```python
from build123d import *

# Parameters (mm, degrees)
SKETCH1_W           = 133
SKETCH1_H           = 105
BOSS_EXTRUDE1_DEPTH = 60
CUT_EXTRUDE1_START  = -2
CUT_EXTRUDE1_DEPTH  = 129
SKETCH3_R           = 42.5
CUT_EXTRUDE2_DEPTH  = 10
FILLET1_R           = 2.5
SKETCH4_W           = 50
SKETCH4_H           = 45
BOSS_EXTRUDE2_DEPTH = 6
SKETCH5_R           = 2.525
CUT_EXTRUDE3_DEPTH  = 4
BOSS_EXTRUDE3_START = 6.5
BOSS_EXTRUDE3_DEPTH = 5
BOSS_EXTRUDE4_START = 11.5
BOSS_EXTRUDE4_DEPTH = 5
CUT_EXTRUDE5_REACH  = 182.394


with BuildPart() as part:
    # Sketch1 → Boss-Extrude1 (new body)
    with BuildSketch(Plane(origin=(0, 0, 0), x_dir=(1, 0, 0), z_dir=(0, 1, 0))):
        with Locations((66.5, 52.5)):
            Rectangle(SKETCH1_W, SKETCH1_H)
    extrude(amount=BOSS_EXTRUDE1_DEPTH)

    # Sketch2 → Cut-Extrude1 (cut)
    with BuildSketch(Plane.ZY.offset(CUT_EXTRUDE1_START)):
        with BuildLine():
            Line((-99, 0), (-6, 0))
            ThreePointArc((-6, 0), (-52.5, 46.5), (-99, 0))
        make_face()
    extrude(amount=-CUT_EXTRUDE1_DEPTH, mode=Mode.SUBTRACT)

    # Sketch3 → Cut-Extrude2 (cut)
    with BuildSketch(Plane.ZY):
        with Locations((-52.5, 0)):
            Circle(SKETCH3_R)
    extrude(amount=-CUT_EXTRUDE2_DEPTH, mode=Mode.SUBTRACT)

    # Fillet1
    # the kernel refuses this fillet: 2.5 mm, written as the material it takes off along each edge
    with BuildSketch(Plane(origin=(130.5, 57.5, -102.5), x_dir=(0, 1, 0), z_dir=(1, 0, 0))) as fillet1_piece_1_section:
        Polygon((0, 0), (FILLET1_R * 1.02, 0), (FILLET1_R * 1.02, -FILLET1_R * 1.02), (0, -FILLET1_R * 1.02), align=None)
    fillet1_piece_1 = extrude(amount=FILLET1_R * 1.02, mode=Mode.PRIVATE)
    fillet1_piece_1 = fillet1_piece_1 - Plane(origin=(130.5, 57.5, -102.5), x_dir=(0, -0.7071067811865475, 0.7071067811865475), z_dir=(1, 0, 0)) * Sphere(FILLET1_R, mode=Mode.PRIVATE)
    add(fillet1_piece_1, mode=Mode.SUBTRACT)
    with BuildSketch(Plane(origin=(2.5, 57.5, -102.5), x_dir=(0, 1, 0), z_dir=(-1, 0, 0))) as fillet1_piece_2_section:
        Polygon((0, 0), (FILLET1_R * 1.02, 0), (FILLET1_R * 1.02, FILLET1_R * 1.02), (0, FILLET1_R * 1.02), align=None)
    fillet1_piece_2 = extrude(amount=FILLET1_R * 1.02, mode=Mode.PRIVATE)
    fillet1_piece_2 = fillet1_piece_2 - Plane(origin=(2.5, 57.5, -102.5), x_dir=(0, -0.7071067811865475, 0.7071067811865475), z_dir=(-1, 0, 0)) * Sphere(FILLET1_R, mode=Mode.PRIVATE)
    add(fillet1_piece_2, mode=Mode.SUBTRACT)
    with BuildSketch(Plane(origin=(130.5, 57.5, -2.5), x_dir=(1, 0, 0), z_dir=(0, 0, 1))) as fillet1_piece_3_section:
        Polygon((0, 0), (FILLET1_R * 1.02, 0), (FILLET1_R * 1.02, FILLET1_R * 1.02), (0, FILLET1_R * 1.02), align=None)
    fillet1_piece_3 = extrude(amount=FILLET1_R * 1.02, mode=Mode.PRIVATE)
    fillet1_piece_3 = fillet1_piece_3 - Plane(origin=(130.5, 57.5, -2.5), x_dir=(-0.7071067811865475, -0.7071067811865475, 0), z_dir=(0, 0, 1)) * Sphere(FILLET1_R, mode=Mode.PRIVATE)
    add(fillet1_piece_3, mode=Mode.SUBTRACT)
    with BuildSketch(Plane(origin=(2.5, 57.5, -2.5), x_dir=(-1, 0, 0), z_dir=(0, 0, 1))) as fillet1_piece_4_section:
        Polygon((0, 0), (FILLET1_R * 1.02, 0), (FILLET1_R * 1.02, -FILLET1_R * 1.02), (0, -FILLET1_R * 1.02), align=None)
    fillet1_piece_4 = extrude(amount=FILLET1_R * 1.02, mode=Mode.PRIVATE)
    fillet1_piece_4 = fillet1_piece_4 - Plane(origin=(2.5, 57.5, -2.5), x_dir=(0.7071067811865475, -0.7071067811865475, 0), z_dir=(0, 0, 1)) * Sphere(FILLET1_R, mode=Mode.PRIVATE)
    add(fillet1_piece_4, mode=Mode.SUBTRACT)
    with BuildSketch(Plane(origin=(130.5, 60, -105), x_dir=(0, 0, 1), z_dir=(-1, 0, 0))) as fillet1_piece_5:
        with BuildLine():
            CenterArc((FILLET1_R, -FILLET1_R), FILLET1_R, 90, 90)
            Line((0, -FILLET1_R), (0, 0))
            Line((0, 0), (FILLET1_R, 0))
        make_face()
    extrude(amount=128, mode=Mode.SUBTRACT)
    with BuildSketch(Plane(origin=(133, 60, -2.5), x_dir=(0, -1, 0), z_dir=(0, 0, -1)), Plane(origin=(0, 60, -102.5), x_dir=(0, -1, 0), z_dir=(0, 0, 1))) as fillet1_piece_6:
        with BuildLine():
            CenterArc((FILLET1_R, FILLET1_R), FILLET1_R, 180, 90)
            Line((0, FILLET1_R), (0, 0))
            Line((0, 0), (FILLET1_R, 0))
        make_face()
    extrude(amount=100, mode=Mode.SUBTRACT)
    with BuildSketch(Plane(origin=(2.5, 60, 0), x_dir=(0, -1, 0), z_dir=(1, 0, 0))) as fillet1_piece_7:
        with BuildLine():
            CenterArc((FILLET1_R, FILLET1_R), FILLET1_R, 180, 90)
            Line((0, FILLET1_R), (0, 0))
            Line((0, 0), (FILLET1_R, 0))
        make_face()
    extrude(amount=128, mode=Mode.SUBTRACT)
    with BuildSketch(Plane(origin=(133, -6.25, 0), x_dir=(-1, 0, 0), z_dir=(0, 1, 0)), Plane(origin=(133, -6.25, -105), x_dir=(0, 0, 1), z_dir=(0, 1, 0))) as fillet1_piece_8:
        with BuildLine():
            CenterArc((FILLET1_R, -FILLET1_R), FILLET1_R, 90, 90)
            Line((0, -FILLET1_R), (0, 0))
            Line((0, 0), (FILLET1_R, 0))
        make_face()
    extrude(amount=63.75, mode=Mode.SUBTRACT)
    with BuildSketch(Plane(origin=(133, 0, 6.25), x_dir=(0, 1, 0), z_dir=(0, 0, -1))) as fillet1_piece_9:
        with BuildLine():
            CenterArc((FILLET1_R, -FILLET1_R), FILLET1_R, 90, 90)
            Line((0, -FILLET1_R), (0, 0))
            Line((0, 0), (FILLET1_R, 0))
        make_face()
    extrude(amount=117.5, mode=Mode.SUBTRACT)
    with BuildSketch(Plane(origin=(0, -6.25, -105), x_dir=(0, 0, 1), z_dir=(0, 1, 0)), Plane(origin=(0, -6.25, 0), x_dir=(1, 0, 0), z_dir=(0, 1, 0))) as fillet1_piece_10:
        with BuildLine():
            CenterArc((FILLET1_R, FILLET1_R), FILLET1_R, 180, 90)
            Line((0, FILLET1_R), (0, 0))
            Line((0, 0), (FILLET1_R, 0))
        make_face()
    extrude(amount=63.75, mode=Mode.SUBTRACT)
    with BuildSketch(Plane(origin=(0, 0, -16.25), x_dir=(0, 1, 0), z_dir=(0, 0, 1)), Plane(origin=(0, 0, -111.25), x_dir=(0, 1, 0), z_dir=(0, 0, 1))) as fillet1_piece_11:
        with BuildLine():
            CenterArc((FILLET1_R, -FILLET1_R), FILLET1_R, 90, 90)
            Line((0, -FILLET1_R), (0, 0))
            Line((0, 0), (FILLET1_R, 0))
        make_face()
    extrude(amount=22.5, mode=Mode.SUBTRACT)
    with BuildSketch(Plane(origin=(0, 0, -52.5), x_dir=(0, -0.14381889116089097, 0.9896040251258337), z_dir=(0, -0.9896040251258337, -0.14381889116089097))) as fillet1_piece_12:
        with BuildLine():
            CenterArc((44.949489743, -2.5), FILLET1_R, 90, 78.463040967)
            Line((42.5, -2), (42.5, 0))
            Line((42.5, 0), (44.949489743, 0))
        make_face()
    revolve(axis=Axis((0, 0, -52.5), (-1, 0, 0)), revolution_arc=196.537779553, mode=Mode.SUBTRACT)

    # Sketch4 → Boss-Extrude2 (add)
    with BuildSketch(Plane(origin=(0, 60, 0), x_dir=(1, 0, 0), z_dir=(0, 1, 0))):
        with Locations((66.5, 52.5)):
            Rectangle(SKETCH4_W, SKETCH4_H)
    extrude(amount=BOSS_EXTRUDE2_DEPTH)

    # Sketch5 → Cut-Extrude3 (cut)
    with BuildSketch(Plane(origin=(0, 66, 0), x_dir=(1, 0, 0), z_dir=(0, 1, 0))):
        with Locations(Location((47.5, 68.5, 0), (0, 0, 270))):
            Circle(SKETCH5_R)
        with Locations(Location((85.5, 68.5, 0), (0, 0, 270))):
            Circle(SKETCH5_R)
        with Locations(Location((85.5, 36.5, 0), (0, 0, 270))):
            Circle(SKETCH5_R)
        with Locations(Location((47.5, 36.5, 0), (0, 0, 270))):
            Circle(SKETCH5_R)
    extrude(amount=-CUT_EXTRUDE3_DEPTH, mode=Mode.SUBTRACT)

    # Sketch6 → Boss-Extrude3 (add)
    with BuildSketch(Plane(origin=(2, 0, 0), x_dir=(0, 0, -1), z_dir=(1, 0, 0)).offset(BOSS_EXTRUDE3_START)):
        with BuildLine():
            Line((94.999969985, 0.050510257), (98.999972567, 0.050510257))
            ThreePointArc((98.999972567, 0.050510257), (52.5, 46.5), (6.000027433, 0.050510257))
            Line((6.000027433, 0.050510257), (10.000030015, 0.050510257))
            ThreePointArc((10.000030015, 0.050510257), (52.5, 42.5), (94.999969985, 0.050510257))
        make_face()
    extrude(amount=BOSS_EXTRUDE3_DEPTH)

    # Sketch7 → Boss-Extrude4 (add)
    with BuildSketch(Plane.ZY.offset(-131).offset(BOSS_EXTRUDE4_START)):
        with BuildLine():
            Line((-6.000027433, 0.050510257), (-10.000030015, 0.050510257))
            ThreePointArc((-10.000030015, 0.050510257), (-52.5, 42.5), (-94.999969985, 0.050510257))
            Line((-94.999969985, 0.050510257), (-98.999972567, 0.050510257))
            ThreePointArc((-98.999972567, 0.050510257), (-52.5, 46.5), (-6.000027433, 0.050510257))
        make_face()
    extrude(amount=-BOSS_EXTRUDE4_DEPTH)

    # Cut-Extrude5: up to this face of the body (flat: up to its plane)
    cut_extrude5_end = Plane(part.part.faces().sort_by_distance((131, 19.762510478, -52.5))[0])
    # Sketch14 → Cut-Extrude5 (cut, up to the picked face)
    with BuildSketch(Plane.ZY.offset(-2), mode=Mode.PRIVATE) as cut_extrude5_sk1:
        with BuildLine():
            Line((-22.531752229, 44.110383395), (-18.996218323, 47.645917301))
            Line((-18.996218323, 47.645917301), (-4.854082699, 33.503781677))
            Line((-4.854082699, 33.503781677), (-8.389616605, 29.968247771))
            ThreePointArc((-8.389616605, 29.968247771), (-10.100706376, 23.286397782), (-9.016282965, 16.474718596))
            Line((-9.016282965, 16.474718596), (-12.593550728, 14.619346994))
            ThreePointArc((-12.593550728, 14.619346994), (-22.4479618, 30.0520382), (-37.880653006, 39.906449272))
            Line((-37.880653006, 39.906449272), (-36.025281404, 43.483717035))
            ThreePointArc((-36.025281404, 43.483717035), (-29.213602218, 42.399293624), (-22.531752229, 44.110383395))
        make_face()
    cut_extrude5_tool1 = split(extrude(cut_extrude5_sk1.sketch, amount=-CUT_EXTRUDE5_REACH, mode=Mode.PRIVATE), bisect_by=cut_extrude5_end, keep=Keep.BOTH, mode=Mode.PRIVATE)
    cut_extrude5 = cut_extrude5_tool1.solids().sort_by(Axis((2, 34.053009, -18.446991), (1, 0, 0)))[0]
    add(cut_extrude5, mode=Mode.SUBTRACT)

    # Mirror3: Cut-Extrude5 across plane
    add(cut_extrude5.mirror(Plane(origin=(0, 0, -52.5), x_dir=(1, 0, 0), z_dir=(0, 0, -1))), mode=Mode.SUBTRACT)


solid = part.part
```
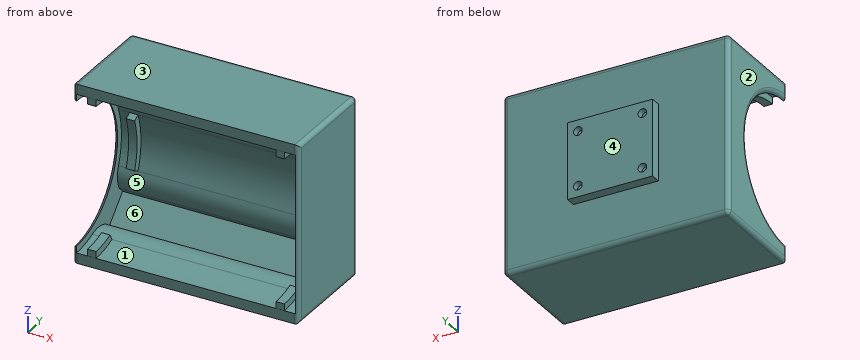
Verification items for the finished model (mm, model axes). Face numbers are marked on the shaded views. A direction names the side the tool comes from. Coordinates: 2 decimals unless noted, no trailing zeros. Write each loop counter-clockwise with the first axis right and the second up, starting at its lowest first coordinate (ties: lowest second). Pieces come first, ordered by that corner, then holes. Notation, with made-up numbers: (-33, 66) - (-14, 66) arc R31 cw to (-14, 105) - close; hole circle Ø9 at (56, 31). An arc over 180 degrees is marked (long way). Write item = value, one per line.
Q1. Mould release check, pull along Z, two halves, no side actions. Record for the marked faces 3, 4, 5 and 6: released by +Z, released by -Z, zero draft, split by the parting line, or undercut.
Answer:
face_3 = released by +Z
face_4 = zero draft
face_5 = undercut
face_6 = undercut
Q2. Material ranges on L1, parallel to X at y = 64.95, z = -68.5 (3 decimals); L2, parallel to X at y = 46, z = -53; L3, parallel to Z at x = 85, y = 64 (3 decimals), recorded low to high. Write a range as from..to.
Answer:
L1 = 41.5..44.975, 50.025..82.975, 88.025..91.5
L2 = 0..2, 8.5..13.5, 119.5..124.5, 131..133
L3 = -75..-70.975, -66.025..-38.975, -34.025..-30
Q3. Access from +Z, -Z, +X, -X, +Y, -Y to the whole of each face (thin tool, end or side, straight path). Record for the marked faces 1 and 2.
Answer:
face_1 = -Y
face_2 = +Z, -Z, -X, +Y, -Y
Q4. Cross-section at B-B (x = 111.5). Enter the section's corners in (y, z).
Answer:
outline = (0, -105) - (57.5, -105) arc R2.5 ccw to (60, -102.5) - (60, -2.5) arc R2.5 ccw to (57.5, 0) - (0, 0) - (0, -6) arc R46.5 cw to (16.47, -9.02) arc R17 ccw to (29.97, -8.39) - (33.5, -4.85) - (47.65, -19) - (44.11, -22.53) arc R17 ccw to (43.48, -36.03) arc R46.5 cw to (43.48, -68.97) arc R17 ccw to (44.11, -82.47) - (47.65, -86) - (33.5, -100.15) - (29.97, -96.61) arc R17 ccw to (16.47, -95.98) arc R46.5 cw to (0, -99) - close
Q5. Go/stop test with flat-tipped pins: pin 1 Ø3.5 at (y, z) = (11.5, -96) entering from -X; pin 2 Ø2 at (x, z) = (11, -9) entering from -Y; pin 3 Ø8 at (x, z) = (110.5, -53) entering from +Y; pin 4 Ø2.5 at (x, z) = (47, -67.5) entering from +Y. Record where each tip stops, or that it passes through.
Answer:
pin_1 = 0
pin_2 = 0.05
pin_3 = 60
pin_4 = 62
Q6. Cross-section at C-C (x = 63.5). Enter the section's corners in (y, z), plus the area to 3 significant figures.
Answer:
outline = (0, -105) - (57.5, -105) arc R2.5 ccw to (60, -102.5) - (60, -75) - (66, -75) - (66, -30) - (60, -30) - (60, -2.5) arc R2.5 ccw to (57.5, 0) - (0, 0) - (0, -6) arc R46.5 cw to (16.47, -9.02) arc R17 ccw to (29.97, -8.39) - (33.5, -4.85) - (47.65, -19) - (44.11, -22.53) arc R17 ccw to (43.48, -36.03) arc R46.5 cw to (43.48, -68.97) arc R17 ccw to (44.11, -82.47) - (47.65, -86) - (33.5, -100.15) - (29.97, -96.61) arc R17 ccw to (16.47, -95.98) arc R46.5 cw to (0, -99) - close
area = 2,650 mm²
